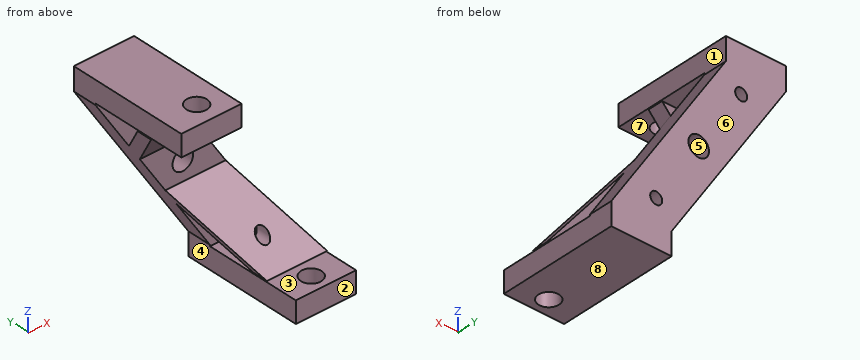
from build123d import *
from build123d.topology import SkipClean

# Parameters (mm, degrees)
SCHIZZO9_W                          = 10
SCHIZZO9_H                          = 20
ESTRUSIONE_ESTRUSIONE5_DEPTH        = 35.05
SCHIZZO10_W                         = 35.05
SCHIZZO10_H                         = 16
TAGLIO_ESTRUSIONE1_DEPTH            = 43.05
SCHIZZO11_R                         = 1.7
TAGLIO_ESTRUSIONE2_DEPTH            = 43.05
SCHIZZO16_W                         = 10
SCHIZZO16_H                         = 4
ESTRUSIONE_ESTRUSIONE8_DEPTH        = 4
SCHIZZO17_W                         = 10
SCHIZZO17_H                         = 4
ESTRUSIONE_ESTRUSIONE9_DEPTH        = 4
ESTRUSIONE_ESTRUSIONE10_OUTLINE_W   = 10
ESTRUSIONE_ESTRUSIONE10_OUTLINE_H   = 3.78
ESTRUSIONE_ESTRUSIONE10_OUTLINE_H_2 = 3.75
ESTRUSIONE_ESTRUSIONE10_DEPTH       = 16
ESTRUSIONE_ESTRUSIONE11_DEPTH       = 10.000000119
ESTRUSIONE_ESTRUSIONE12_DEPTH       = 10.000000119
SCHIZZO21_R                         = 1.7
TAGLIO_ESTRUSIONE5_DEPTH            = 4
TAGLIO_ESTRUSIONE7_DEPTH            = 49.638074625
TAGLIO_ESTRUSIONE7_DEPTH_BACK       = 49.638074625
SCHIZZO23_R                         = 1
TAGLIO_ESTRUSIONE8_DEPTH            = 49.638074625
TAGLIO_ESTRUSIONE8_DEPTH_BACK       = 49.638074625
SCHIZZO24_W                         = 10
SCHIZZO24_H                         = 0.25
SCHIZZO24_H_2                       = 0.22
SCHIZZO25_R                         = 1.7
TAGLIO_ESTRUSIONE9_DEPTH            = 10


# Read off the part's stored shape, not the designer's step: Estrusione-Estrusione10
with BuildPart() as part:
    # Schizzo9 → Estrusione-Estrusione5 (new, along a direction that is not the sketch's normal)
    with BuildSketch(Plane.XY):
        with Locations((5, -10)):
            Rectangle(SCHIZZO9_W, SCHIZZO9_H)
    extrude(amount=-ESTRUSIONE_ESTRUSIONE5_DEPTH, dir=(-0.5415393694615634, 0, 0.8406753899830615))

    # Schizzo10 → Taglio-Estrusione1 (cut, along a direction that is not the sketch's normal)
    with BuildSketch(Plane(origin=(7.067351113, 0, 4.552588206), x_dir=(0.5415393694615636, 0, -0.8406753899830613), z_dir=(0.8406753899830615, 0, 0.5415393694615636))):
        with Locations((22.940393695, -12)):
            Rectangle(SCHIZZO10_W, SCHIZZO10_H)
    extrude(amount=-TAGLIO_ESTRUSIONE1_DEPTH, dir=(1, 0, 0), mode=Mode.SUBTRACT)

    # Schizzo11 → Taglio-Estrusione2 (cut)
    with BuildSketch(Plane(origin=(0, 0, 0), x_dir=(1, 0, 0), z_dir=(0, 1, 0))):
        with Locations(Location((14.49047745, 14.732836209, 0), (0, 0, 270))):
            Circle(SCHIZZO11_R)
    extrude(amount=-TAGLIO_ESTRUSIONE2_DEPTH, mode=Mode.SUBTRACT)

    # Schizzo16 → Estrusione-Estrusione8 (add)
    with BuildSketch(Plane(origin=(0, 0, -29.465672419), x_dir=(-1, 0, 0), z_dir=(0, 0, -1))):
        with Locations((-23.9809549, -2)):
            Rectangle(SCHIZZO16_W, SCHIZZO16_H)
    extrude(amount=ESTRUSIONE_ESTRUSIONE8_DEPTH)

    # Schizzo17 → Estrusione-Estrusione9 (add)
    with BuildSketch(Plane.XY):
        with Locations((5, -2)):
            Rectangle(SCHIZZO17_W, SCHIZZO17_H)
    extrude(amount=ESTRUSIONE_ESTRUSIONE9_DEPTH)

    # Estrusione-Estrusione10 outline → Estrusione-Estrusione10 (add)
    with BuildSketch(Plane.XZ.offset(4)):
        with Locations((23.9809549, -31.575672419)):
            Rectangle(ESTRUSIONE_ESTRUSIONE10_OUTLINE_W, ESTRUSIONE_ESTRUSIONE10_OUTLINE_H)
        with Locations((5, 2.125)):
            Rectangle(ESTRUSIONE_ESTRUSIONE10_OUTLINE_W, ESTRUSIONE_ESTRUSIONE10_OUTLINE_H_2)
    extrude(amount=ESTRUSIONE_ESTRUSIONE10_DEPTH)

    # Schizzo19 → Estrusione-Estrusione11 (add, along a direction that is not the sketch's normal)
    with BuildSketch(Plane(origin=(0, 0, 0), x_dir=(-0.5415393694615636, 0, 0.8406753899830613), z_dir=(-0.8406753899830615, 0, -0.5415393694615636))):
        Polygon((-35.234948586, -12), (-24.717369686, -4), (-21.413778213, -4), (-35.234948586, -14.512815167), align=None)
    extrude(amount=-ESTRUSIONE_ESTRUSIONE11_DEPTH, dir=(-1, 0, 0))

    # Schizzo20 → Estrusione-Estrusione12 (add, along a direction that is not the sketch's normal)
    with SkipClean():  # the faces are left unmerged after this step: merging them gives an invalid solid
        with BuildSketch(Plane(origin=(0, 0, 0), x_dir=(-0.5415393694615636, 0, 0.8406753899830613), z_dir=(-0.8406753899830615, 0, -0.5415393694615636))):
            Polygon((0.210168847, -12), (-10.307410052, -4), (-13.611001525, -4), (0.210168847, -14.512815167), align=None)
        extrude(amount=-ESTRUSIONE_ESTRUSIONE12_DEPTH, dir=(-1, 0, 0))

    # Schizzo21 → Taglio-Estrusione5 (cut)
    with SkipClean():  # the faces are left unmerged after this step: merging them gives an invalid solid
        with BuildSketch(Plane.XY.offset(-29.685672419)):
            with Locations((23.9809549, -17.25)):
                Circle(SCHIZZO21_R)
        extrude(amount=-TAGLIO_ESTRUSIONE5_DEPTH, mode=Mode.SUBTRACT)

    # Schizzo23 → Taglio-Estrusione7 (cut, two sides: drawn at the far end of the back side and taken through both)
    with SkipClean():  # the faces are left unmerged after this step: merging them gives an invalid solid
        with BuildSketch(Plane(origin=(0, 0, 0), x_dir=(1, 0, 0), z_dir=(0, 1, 0)).offset(-TAGLIO_ESTRUSIONE7_DEPTH_BACK)):
            with Locations(Location((7.453304803, 3.802227757, 0), (0, 0, 90))):
                Circle(SCHIZZO23_R)
            with Locations(Location((21.533327934, 25.659787159, 0), (0, 0, 270))):
                Circle(SCHIZZO23_R)
        extrude(amount=TAGLIO_ESTRUSIONE7_DEPTH + TAGLIO_ESTRUSIONE7_DEPTH_BACK, mode=Mode.SUBTRACT)

    # Schizzo24 → Taglio-Estrusione8 (cut, two sides: drawn at the far end of the back side and taken through both)
    with SkipClean():  # the faces are left unmerged after this step: merging them gives an invalid solid
        with BuildSketch(Plane(origin=(0, 0, 0), x_dir=(1, 0, 0), z_dir=(0, 1, 0)).offset(-TAGLIO_ESTRUSIONE8_DEPTH_BACK)):
            with Locations((23.9809549, 33.340672419)):
                Rectangle(SCHIZZO24_W, SCHIZZO24_H)
            with Locations((5, -3.89)):
                Rectangle(SCHIZZO24_W, SCHIZZO24_H_2)
        extrude(amount=TAGLIO_ESTRUSIONE8_DEPTH + TAGLIO_ESTRUSIONE8_DEPTH_BACK, mode=Mode.SUBTRACT)

    # Schizzo25 → Taglio-Estrusione9 (cut)
    with SkipClean():  # the faces are left unmerged after this step: merging them gives an invalid solid
        with BuildSketch(Plane.XY.offset(3.78)):
            with Locations((5.741708588, -16.417479931)):
                Circle(SCHIZZO25_R)
        extrude(amount=-TAGLIO_ESTRUSIONE9_DEPTH, mode=Mode.SUBTRACT)


solid = part.part
Can you work these out from the model? Positions are in its coordinate system, mm. Face numbers are marked on the shaded views. A direction names the side the tool comes from. Round coordinates to 2 decimals unless told otherwise and drop trailing zeros. Loops run counter-clockwise (first coordinate to the right, second up) from the corner with the lowest first, then second, coordinate; pieces in that order, holes last. Notation, with made-up numbers: (52.5, -37.5) - (83.5, -37.5) arc R22 cw to (83.5, -0.5) - close; hole circle Ø2 at (19, -13.5). An arc over 180 degrees is marked (long way). Answer in a Markdown table with one row per item. Add a question column.
Q1. I need wall thicknesses on L1, parallel to X at y = -16.25, z = 2; L2, parallel to Z at x = 24.5, y = -8.25; L3, parallel to Y at x = 23.75, z = -29. Which ranges of each line are inside material? Lowest first, please.
Q2. I want a section at C-C on x = 3.5. List the corners of the cut face in (y, z) for me, and give its area (3 significant figures).
Q3. For pin 1 Ø1.9 at (y, z) = (-7.5, 2.5) entering from +X; pin 2 Ø8 at (y, z) = (-9.5, -21.5) entering from +X; pin 3 Ø3.5 at (x, z) = (13.5, -14) entering from -Y, each with a flat end and sliding along its axis, tell me the tip position at first contact or that it passes through.
Q4. I want a section at A-A on y = -9.5. List the corners of the cut face in (x, z) for me.
Q5. Which directions (+Z, -Z, +X, -X, +Y, -Y) give clear straight access to the entire face, cutting with the end or side of a thin tool? Please do the marked faces 1, 2, 3, 4 and 5.
Q6. I want a section at B-B on z = -0.5. List the corners of the cut face in (x, y) for me.
Q7. I want a section at D-D on y = -17.25. List the corners of the cut face in (x, z) for me, and give its area (3 significant figures).
Q8. We'd pull the mould along Z, two halves only. Please class the marked faces 6, 7 and 8: pulls with the +Z half, pulls with the -Z half, needs draft (parallel to the pull), parting line crosses it, or undercut.
A:
| question | item | result |
|---|---|---|
| 1 | L1 | 0 to 4.05, 7.43 to 10 |
| 1 | L2 | -33.22 to -29.69, -25.48 to -22.7 |
| 1 | L3 | -13.95 to -11.44, -4 to 0 |
| 2 | outline | (-20, 0.25) - (-4, 0.25) - (-4, -5.43) - (0, -5.43) - (0, 3.78) - (-20, 3.78) - close; (-14.51, 0.18) - (-9.44, -5.43) - (-6.92, -5.43) - (-12, 0.18) - close |
| 2 | area | 107 mm^2 |
| 3 | pin 1 | x = 10 |
| 3 | pin 2 | x = 26.43 |
| 3 | pin 3 | y = -4 |
| 4 | outline | (0, 0.25) - (10, 0.25) - (10, 3.78) - (0, 3.78) - close; (1.67, -2.59) - (3.46, -5.36) - (13.46, -5.36) - (11.67, -2.59) - close; (15.51, -24.08) - (17.3, -26.86) - (27.3, -26.86) - (25.51, -24.08) - close; (18.98, -33.22) - (28.98, -33.22) - (28.98, -29.69) - (18.98, -29.69) - close; hole circle Ø2 at (7.45, -3.8); hole circle Ø2 at (21.53, -25.66) |
| 5 | face 1 | +Z, +X, +Y, -Y |
| 5 | face 2 | +Z, -Z, +X, -X, -Y |
| 5 | face 3 | +X, -X, -Y |
| 5 | face 4 | -Z, -X, +Y, -Y |
| 5 | face 5 | +Y, -Y |
| 6 | outline | (0.32, -13.9) - (10.32, -13.9) - (10.32, -11.39) - (0.32, -11.39) - close; (0.32, -4) - (10.32, -4) - (10.32, 0) - (0.32, 0) - close |
| 7 | outline | (0, 0.25) - (4.26, 0.25) - (4.26, 3.78) - (0, 3.78) - close; (7.22, 0.25) - (10, 0.25) - (10, 3.78) - (7.22, 3.78) - close; (18.98, -33.22) - (22.28, -33.22) - (22.28, -29.69) - (18.98, -29.69) - close; (25.68, -33.22) - (28.98, -33.22) - (28.98, -29.69) - (25.68, -29.69) - close |
| 7 | area | 48.1 mm^2 |
| 8 | face 6 | needs draft |
| 8 | face 7 | undercut |
| 8 | face 8 | pulls with the -Z half |
